Check sheet for the modelled part. Datum: model origin and axes. Units: mm. A direction names the side the tool comes from. Round coordinates to 2 decimals unless told otherwise and drop trailing zeros. Loops run counter-clockwise (first coordinate to the right, second up) from the corner with the lowest first, then second, coordinate; pieces in that order, holes last. Notation, with made-up numbers: (10.5, 75) - (67.5, 75) arc R25 ccw to (67.5, 105) - close; hole circle Ø4 at (8, 46.5). An arc over 180 degrees is marked (long way). Answer in a Markdown table with one row per item. Add a question column.
(1) Thickness scan on line 1 along Y through (x, z) = (44.5, 0); line 2 along Z through (x, y) = (22, 6.25); line 3 along X through (y, z) = (0.5, 1). Record the ranges inside material, lowest first.
(2) Cross-section at A-A on z = 0. Enter the section's corners in (x, y).
(3) Mould release check, pull along X, two halves, no side actions. Record for faces 1 (the flat face through (-36, 10, 0)), 2 (the flat face through (56, 5, -6)), 3 (the flat face through (42, 5, -2)): +X half, -X half, draft (parallel to the pull), parting line (faces both ways), or undercut.
(4) Gauge pin test, flat ends, axial feed: pin 1 (2.5 mm diameter, centred on y = 7, z = 2, fed in from +X); pin 2 (3 mm diameter, centred on y = 6, z = 1.5, fed in from -X); pin 3 (0.7 mm diameter, centred on x = -51.5, z = -8.5, fed in from +Y). Record the tip position at first contact, or that the pin passes through.
(5) Cross-section at D-D on x = -20.5. Enter the section's corners in (y, z).
(6) Cross-section at B-B on x = 35.5. Enter the section's corners in (y, z), then the cut area to 3 significant figures.
(7) Access from +Z, -Z, +X, -X, +Y, -Y to the whole of each face (thin tool, end or side, straight path). Record for faces 4 (the flat face through (-95, 5, 0)), 5 (the cylindrical face through (-95.1, 9.17, 6.64)), 6 (the flat face through (17, 5, -3.122)), 7 (the cylindrical face through (-95.14, 9.17, -6.6)).
(8) Cross-section at C-C on y = 5. Enter the section's corners in (x, z).
Autodesk Inventor part; units mm, degrees
ref_plane "Plano de trabajo1" through (-95, 5, 4.5) normal (0, 1, 0) x (1, 0, 0)
ref_plane "YZ Plane" through (0, 0, 0) normal (1, 0, 0) x (0, 1, 0)
ref_plane "XZ Plane" through (0, 0, 0) normal (0, 1, 0) x (-1, 0, 0)
sketch "Boceto1" plane through (0, 0, 0) normal (0, 1, 0) x (-1, 0, 0)
  line L0 (96, 7.5) -> (-96, 7.5)
  line L1 (-96, 7.5) -> (-96, -7.5)
  line L2 (-96, -7.5) -> (96, -7.5)
  line L3 (96, -7.5) -> (96, 7.5)
  line L4 (96, 7.5) -> (-96, -7.5) construction
  line L5 (-96, 7.5) -> (96, -7.5) construction
  point P0 (0, 0)
  dimension "d0" = 192
  dimension "d1" = 15
extrude "Extrusión1" add sketch "Boceto1" along normal blind 10
sketch "Boceto2" plane through (0, 0, 0) normal (1, 0, 0) x (0, 1, 0)
  line L0 (0, 7.5) -> (10, 7.5)
  line L1 (2.1, 7.5) -> (7.9, 7.5)
  line L2 (7.9, 7.5) -> (7.9, 9.5)
  line L3 (7.9, 9.5) -> (2.1, 9.5)
  line L4 (2.1, 9.5) -> (2.1, 7.5)
  line L5 (0, -7.5) -> (0, 7.5)
  line L6 (0, -7.5) -> (10, -7.5)
  line L7 (2.1, -7.5) -> (7.9, -7.5)
  line L8 (7.9, -7.5) -> (7.9, -9.5)
  line L9 (7.9, -9.5) -> (2.1, -9.5)
  line L10 (2.1, -9.5) -> (2.1, -7.5)
  point P0 (0, 0)
  point P1 (7.9, -7.5)
  dimension "d4" = 5.8
  dimension "d5" = 2.1
  dimension "d6" = 2
extrude "Extrusión2" add sketch "Boceto2" along normal mid plane 192
sketch "Boceto4" plane through (-96, 0, -7.5) normal (-1, 0, 0) x (0, 0, 1)
  line L0 (15, 2.1) -> (17, 2.1)
  line L1 (0, 7.9) -> (-2, 7.9)
  line L2 (17, 2.1) -> (-2, 2.1)
  line L3 (-2, 2.1) -> (-2, 7.9)
  line L4 (-2, 7.9) -> (17, 7.9)
  line L5 (17, 7.9) -> (17, 2.1)
  point P0 (7.5, 0)
extrude "Extrusión3" cut sketch "Boceto4" against normal blind 1
sketch "Boceto5" plane through (96, 0, 7.5) normal (1, 0, 0) x (0, 0, -1)
  line L0 (0, 7.9) -> (-2, 7.9)
  line L1 (17, 2.1) -> (17, 7.9)
  line L2 (-2, 7.9) -> (17, 7.9)
  line L3 (17, 7.9) -> (17, 2.1)
  line L4 (17, 2.1) -> (-2, 2.1)
  line L5 (-2, 2.1) -> (-2, 7.9)
  point P0 (7.5, 0)
extrude "Extrusión4" cut sketch "Boceto5" against normal blind 1
fillet "Empalme1" radius 5 4 edges at (95, 5, -9.5) (95, 5, 9.5) (-95, 5, -9.5) (-95, 5, 9.5)
fillet "Empalme2" radius 3 8 edges at (96, 8.95, 7.5) (96, 1.05, 7.5) (96, 8.95, -7.5) (96, 1.05, -7.5) (-96, 1.05, 7.5) (-96, 8.95, 7.5) (-96, 1.05, -7.5) (-96, 8.95, -7.5)
sketch "Boceto7" plane through (0, 10, 0) normal (0, 1, 0) x (1, 0, 0)
  line L0 (-90, 9.5) -> (90, 9.5)
  line L1 (-90, -9.5) -> (90, -9.5)
  line L2 (82.6935, 4) -> (-107.9962, 4)
  line L3 (-107.9962, 4) -> (-107.9962, -4)
  line L4 (-107.9962, -4) -> (82.6935, -4)
  line L5 (82.6935, -4) -> (82.6935, 4)
  line L6 (93, 7.5) -> (-93, 7.5)
  line L7 (96, 9.5) -> (66, 9.5)
  line L8 (66, 9.5) -> (66, -22.8831)
  line L9 (66, -22.8831) -> (96, -22.8831)
  line L10 (96, -22.8831) -> (96, 9.5)
  line L11 (96, -4.5) -> (96, 4.5)
  line L12 (66, 9.5) -> (56, 9.5)
  line L13 (56, 9.5) -> (56, 4)
  line L14 (56, 4) -> (66, 4)
  line L15 (66, 4) -> (66, 9.5)
  line L16 (66, -9.5) -> (56, -9.5)
  line L17 (56, -9.5) -> (56, -4)
  line L18 (56, -4) -> (66, -4)
  line L19 (66, -4) -> (66, -9.5)
  line L20 (66, 4) -> (46, 4)
  line L21 (46, 4) -> (46, -4)
  line L22 (46, -4) -> (66, -4)
  line L23 (66, -4) -> (66, 4)
  point P0 (90, 9.5)
  point P1 (66, 4)
  point P2 (66, -4)
  dimension "d17" = 8
  dimension "d18" = 3.5
  dimension "d19" = 30
  dimension "d20" = 10
  dimension "d23" = 10
extrude "Extrusión5" cut sketch "Boceto7" against normal through all contours L0 L8 L6 L13 | L0 L7 L10 L9 L8 L4 L5 L2 | L6 L8 L2 L13 | L2 L8 L4 L21 | L2 L5 L4 L8 | L8 L1 L17 L4
sketch "Boceto8" plane through (0, 10, 0) normal (0, 1, 0) x (1, 0, 0)
  line L0 (56, -0.8) -> (56, -7.5)
  line L1 (46, 4.15) -> (56, 4.15)
  line L2 (56, 4.15) -> (56, -4.15)
  line L3 (56, -4.15) -> (46, -4.15)
  line L4 (46, -4.15) -> (46, 4.15)
  line L5 (46, -4) -> (46, 4)
  line L6 (46, 4) -> (56, 4)
  line L7 (56, -4) -> (46, -4)
  point P0 (0, 0)
  dimension "d24" = 0.15
  dimension "d25" = 0.15
extrude "Extrusión6" cut sketch "Boceto8" against normal through all
sketch "Boceto10" plane through (46, 10, 4.15) normal (1, 0, 0) x (0, 0, -1)
  circle A0 centre (4.15, -5) radius 1.7
  line L0 (8.3, -10) -> (0, -10)
  point P0 (4.15, -10)
  point P1 (4.15, -10)
  dimension "d35" = 3.4
  dimension "d36" = 5
extrude "Extrusión8" cut sketch "Boceto10" against normal blind 7.5
sketch "Boceto11" plane through (0, 10, 0) normal (0, 1, 0) x (1, 0, 0)
  line L0 (-8, -2.8775) -> (42, -2.8775)
  line L1 (42, -2.8775) -> (42, 3.1225)
  line L2 (42, 3.1225) -> (-8, 3.1225)
  line L3 (-8, 3.1225) -> (-8, -2.8775)
  line L4 (46, -4.15) -> (46, 4.15)
  point P0 (0, 0)
  dimension "d39" = 6
  dimension "d40" = 50
  dimension "d41" = 4
extrude "Extrusión9" cut sketch "Boceto11" against normal through all
ref_plane "Plano de trabajo1" through (-95, 5, 4.5) normal (0, 1, 0) x (1, 0, 0)
sketch "Boceto12" plane through (-95, 5, 4.5) normal (0, 1, 0) x (1, 0, 0)
  arc A0 (0.8333, 11.7639) -> (-1, 9) centre (2, 9) ccw
  arc A1 (0.8333, 11.7639) -> (0, 9) centre (5, 9) ccw
  line L0 (0, 9) -> (0, 0)
  arc A2 (0, 0) -> (0.8333, -2.7639) centre (5, 0) ccw
  arc A3 (-1, 0) -> (0.8333, -2.7639) centre (2, 0) ccw
  line L1 (-1, 9) -> (-1, 0)
  point P0 (95, 4.5)
extrude "Extrusión10" cut sketch "Boceto12" along normal mid plane 6.6
sketch "Boceto9" plane through (0, 10, 0) normal (0, 1, 0) x (1, 0, 0)
  line L0 (38.5, 3) -> (42, 3)
  line L1 (42, 3) -> (42, -3)
  line L2 (42, -3) -> (38.5, -3)
  line L3 (38.5, -3) -> (38.5, 3)
  line L4 (38.5, 3) -> (42, -3) construction
  line L5 (42, 3) -> (38.5, -3) construction
  line L6 (46, -4.15) -> (46, 4.15)
  line L7 (42, 1.75) -> (46, 1.75)
  line L8 (46, 1.75) -> (46, -1.75)
  line L9 (46, -1.75) -> (42, -1.75)
  line L10 (42, -1.75) -> (42, 1.75)
  point P0 (0, 0)
  point P1 (40.25, 0)
  dimension "d28" = 6
  dimension "d29" = 3.5
  dimension "d30" = 1.75
  dimension "d31" = 3.5
  dimension "d32" = 4
properties part number "GT2RackA" material "UHMW, negro"
Answers:
| question | item | result |
|---|---|---|
| 1 | line 1 | y = 0 to 3.3, 6.7 to 10 |
| 1 | line 2 | z = -9.5 to -3.12, 2.88 to 9.5 |
| 1 | line 3 | x = -96 to -8, 42 to 46 |
| 2 | outline | (-96, 0) - (-8, 0) - (-8, 10) - (-96, 10) - (-96, 8.3) - (-95, 8.3) - (-95, 1.7) - (-96, 1.7) - close; (42, 0) - (46, 0) - (46, 3.3) - (42, 3.3) - close; (42, 6.7) - (46, 6.7) - (46, 10) - (42, 10) - close |
| 3 | face 1 | draft |
| 3 | face 2 | +X half |
| 3 | face 3 | undercut |
| 4 | pin 1 | stops at x = 46 |
| 4 | pin 2 | stops at x = -95 |
| 4 | pin 3 | stops at y = 7.9 |
| 5 | outline | (0, -7.5) - (2.1, -7.5) - (2.1, -9.5) - (7.9, -9.5) - (7.9, -7.5) - (10, -7.5) - (10, 7.5) - (7.9, 7.5) - (7.9, 9.5) - (2.1, 9.5) - (2.1, 7.5) - (0, 7.5) - close |
| 6 | outline | (0, -7.5) - (2.1, -7.5) - (2.1, -9.5) - (7.9, -9.5) - (7.9, -7.5) - (10, -7.5) - (10, -3.12) - (0, -3.12) - close; (0, 2.88) - (10, 2.88) - (10, 7.5) - (7.9, 7.5) - (7.9, 9.5) - (2.1, 9.5) - (2.1, 7.5) - (0, 7.5) - close |
| 6 | area | 113 mm^2 |
| 7 | face 4 | +Z, -Z, -X |
| 7 | face 5 | +Z, -X, +Y |
| 7 | face 6 | +Y, -Y |
| 7 | face 7 | -Z, -X, +Y |
| 8 | outline | (-95, -4.5) arc R5 ccw to (-90, -9.5) - (56, -9.5) - (56, -4.15) - (46, -4.15) - (46, -1.7) - (42, -1.7) - (42, -3.12) - (-8, -3.12) - (-8, 2.88) - (42, 2.88) - (42, 1.7) - (46, 1.7) - (46, 4.15) - (56, 4.15) - (56, 9.5) - (-90, 9.5) arc R5 ccw to (-95, 4.5) - close |
